Design review of the part built by this model. Coordinates are the model's own, in mm. A direction names the side the tool comes from. Give positions to 0.01 mm unless a question says otherwise; leave off trailing zeros. Order: outer loops, then holes, each group sorted by start corner. A loop starts at its lowest first (then second) coordinate and runs counter-clockwise, first axis right, second up. Notation, with made-up numbers: (53, -40) -> (82, -40) arc R15 ccw to (82, -24) -> close; hole circle Ø3 at (19, 76.25). An arc over 180 degrees is marked (long way). Return JSON: item names as keys, results as strings.
Autodesk Inventor part; units mm, degrees
ref_plane "YZ Plane" through (0, 0, 0) normal (1, 0, 0) x (0, 1, 0)
ref_plane "XZ Plane" through (0, 0, 0) normal (0, 1, 0) x (-1, 0, 0)
ref_plane "XY Plane" through (0, 0, 0) normal (0, 0, 1) x (1, 0, 0)
sketch "Sketch1" plane through (0, 0, 0) normal (0, 0, 1) x (1, 0, 0)
  line L0 (1.3856, 2.4) -> (2.7713, 0)
  line L1 (2.7713, 0) -> (1.3856, -2.4)
  line L2 (1.3856, -2.4) -> (-1.3856, -2.4)
  line L3 (-1.3856, -2.4) -> (-2.7713, 0)
  line L4 (-2.7713, 0) -> (-1.3856, 2.4)
  line L5 (-1.3856, 2.4) -> (1.3856, 2.4)
  point P0 (0, 0)
  dimension "d0" = 4.8
extrude "Extrusion1" add sketch "Sketch1" along normal blind 0.4
sketch "Sketch2" plane through (0, 0, 0.4) normal (0, 0, 1) x (1, 0, 0)
  circle A0 centre (0, 0) radius 2.1
  dimension "d3" = 4.2
extrude "Extrusion2" add sketch "Sketch2" along normal blind 7.6
sketch "Sketch3" plane through (0, 0, 8) normal (0, 0, 1) x (1, 0, 0)
  circle A0 centre (0, 0) radius 2.1
  circle A1 centre (0, 0) radius 1.5
  dimension "d6" = 3
extrude "Extrusion3" cut sketch "Sketch3" against normal blind 10 contours A1
chamfer "Chamfer1" distance 0.3 angle 45 1 edges at (-1.5, 0, 8)
thread "Thread1"
properties part number "Вытяжная заклепка_Р-Ш-М3" material "Сталь низкоуглеродистая"
Item 1: Machinability: for faces 4 (the face through (2.003, -0.631, 4.147)), 5 (the face through (0, 2, 0)), which of the approach directions +Z, -Z, +X, -X, +Y, -Y give a long, thin tool a straight path to every point of the face, cutting with its end or side? Answer none if there is none.
Result set:
{"face 4": "+Z", "face 5": "-Z, +X, -X, +Y, -Y"}
Item 2: Mouldability with a two-part tool opening along X and no side actions: class faces 1 (the face through (2.069, 1.217, 0.197)), 2 (the face through (-1.5, 0.07, 3.9)), 3 (the face through (-2.069, -1.217, 0.197)) as released by +X, released by -X, zero draft, split by the parting line, or undercut.
Result set:
{"face 1": "released by +X", "face 2": "undercut", "face 3": "released by -X"}
Item 3: Wall thickness on L1, parallel to Y at x = 0, z = 3.75; L2, parallel to X at y = -1.25, z = 6.25; L3, parallel to Y at x = -0.65, z = 7: over which ranges is each line inside the solid? List them lowest first. Write a range as [from, to].
Result set:
{"L1": "y = [-2.1, -1.5], [1.5, 2.1]", "L2": "x = [-1.69, -0.83], [0.83, 1.69]", "L3": "y = [-2, -1.35], [1.35, 2]"}
Item 4: For pin 1 (2 mm diameter, centred on x = 1, z = 2, fed in from +Y), flat-tipped, find the tip position at first contact; note if it passes through.
Result set:
{"pin 1": "stops at y = 2.1"}
Item 5: Add section A-A (x = 0). Give the boundary of the cut face in (y, z).
Result set:
{"outline": "(-2.4, 0) -> (-1.5, 0) -> (-1.5, 7.7) -> (-1.8, 8) -> (-2.1, 8) -> (-2.1, 0.4) -> (-2.4, 0.4) -> close; (1.5, 0) -> (2.4, 0) -> (2.4, 0.4) -> (2.1, 0.4) -> (2.1, 8) -> (1.8, 8) -> (1.5, 7.7) -> close"}
Item 6: Add section B-B (z = 2.5). Give the boundary of the cut face in (x, y).
Result set:
{"outline": "circle Ø4.2 at (0, 0); hole circle Ø3 at (0, 0)"}
